Could you check a few things on this drawing? It's one solid part, dimensions in mm from its lowest x, y, z. A direction names the side the tool comes from. Coordinates: 2 decimals unless noted, no trailing zeros. Order: outer loops, then holes, each group sorted by start corner. A loop starts at its lowest first (then second) coordinate and runs counter-clockwise, first axis right, second up.
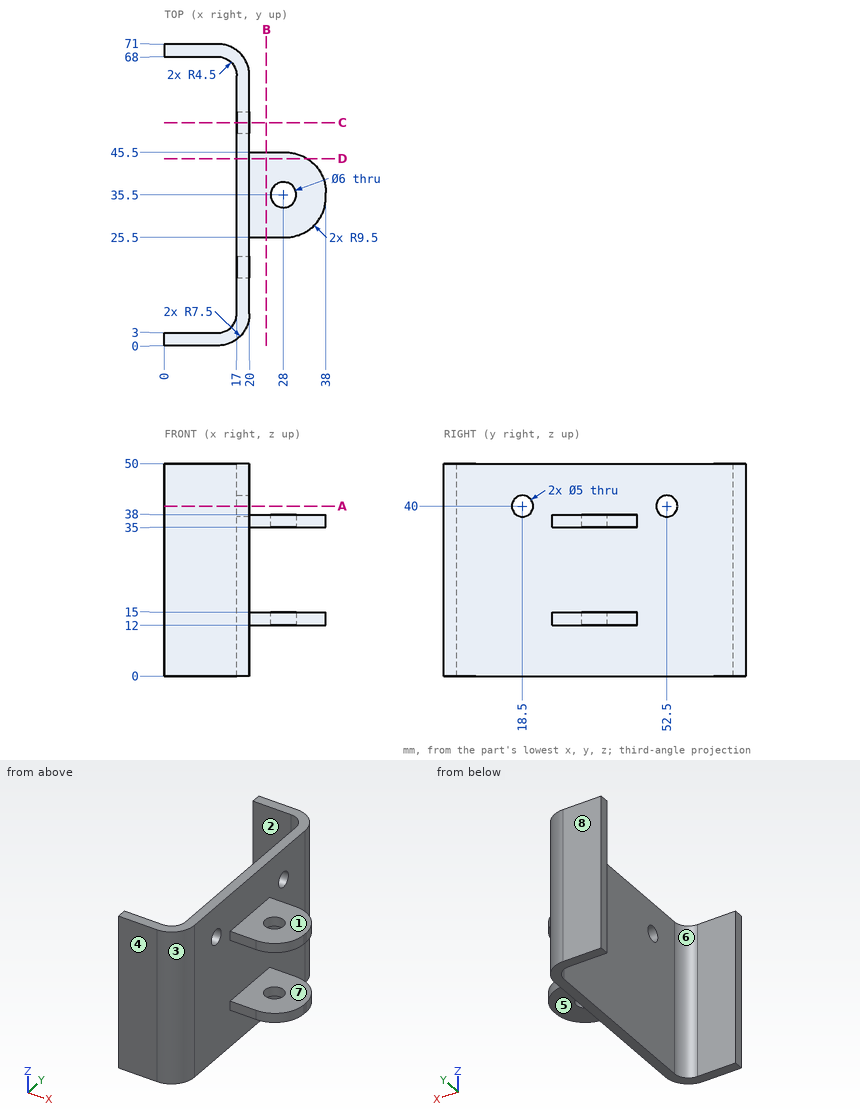
Q1. If we section it at B-B on x = 24: Write out the boundary of the cut face in (y, z).
Q2. If we section it at C-C on y = 52.5: Write out the boundary of the cut face in (x, z).
Q3. If we section it at D-D on y = 44: Write out the boundary of the cut face in (x, z), then the cut area to 3 significant figures.
Q4. We'd pull the mould along Y, two halves only. Please class the marked faces 1, 2 and 3: pulls with the +Y half, pulls with the -Y half, needs draft (parallel to the pull), parting line crosses it, or undercut.
Q5. I need wall thicknesses on L1, parallel to Y at x = 19, z = 40; L2, parallel to Y at x = 18.9, z = 40; L3, parallel to Y at x = 3.5, z = 21. Which ranges of each line are inside material? Lowest first, please.
Q6. For the marked faces 4, 5, 6, 7 and 8, which set-ups out of +Z, -Z, +X, -X, +Y, -Y let a thin tool reach every point of the face, with its end or its side?
Q7. If we section it at A-A on z = 40: Write out the boundary of the cut face in (x, y).
Q8. Will these pins go through, and if not, where does the flat tip stop? pin 1 (1.5 mm diameter, centred on x = 23, z = 36, fed in from +Y); pin 2 (2 mm diameter, centred on x = 16.5, z = 5, fed in from +Y); pin 3 (1 mm diameter, centred on y = 18, z = 37.5, fed in from -X).
Reply:
1. outline: (25.5, 12) - (45.5, 12) - (45.5, 15) - (25.5, 15) - close; (25.5, 35) - (45.5, 35) - (45.5, 38) - (25.5, 38) - close
2. outline: (17, 0) - (20, 0) - (20, 37.5) - (17, 37.5) - close; (17, 42.5) - (20, 42.5) - (20, 50) - (17, 50) - close
3. outline: (17, 0) - (20, 0) - (20, 12) - (33.62, 12) - (33.62, 15) - (20, 15) - (20, 35) - (33.62, 35) - (33.62, 38) - (20, 38) - (20, 50) - (17, 50) - close
3. area: 232 mm2
4. face 1: needs draft
4. face 2: undercut
4. face 3: pulls with the -Y half
5. L1: y = 3.76 to 16, 21 to 50, 55 to 67.24
5. L2: y = 3.59 to 16, 21 to 50, 55 to 67.41
5. L3: y = 0 to 3, 68 to 71
6. face 4: +Z, -Z, +X, -X, -Y
6. face 5: -Z, +X, +Y, -Y
6. face 6: +Z, -Z, -X
6. face 7: +X, +Y, -Y
6. face 8: +Z, -Z, +X, -X, +Y
7. outline: (0, 0) - (12.5, 0) arc R7.5 ccw to (20, 7.5) - (20, 16) - (17, 16) - (17, 7.5) arc R4.5 cw to (12.5, 3) - (0, 3) - close; (0, 68) - (12.5, 68) arc R4.5 cw to (17, 63.5) - (17, 55) - (20, 55) - (20, 63.5) arc R7.5 ccw to (12.5, 71) - (0, 71) - close; (17, 21) - (20, 21) - (20, 50) - (17, 50) - close
8. pin 1: stops at y = 45.5
8. pin 2: stops at y = 70.37
8. pin 3: stops at x = 17
